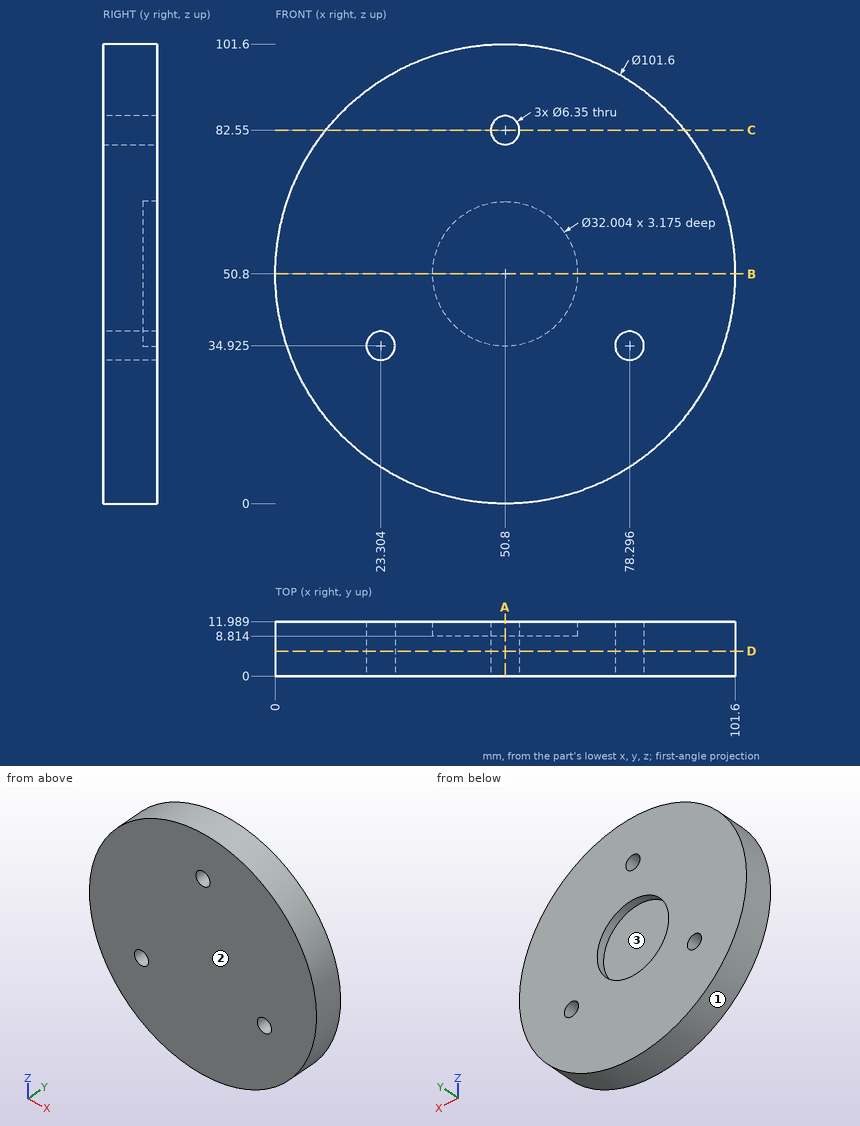
Geometry: see drawing. Coordinates: mm, zero at the bounding-box minimum. Give positions to 0.01 mm unless a question says otherwise; leave off trailing zeros. Order: outer loops, then holes, each group sorted by start corner. A loop starts at its lowest first (then second) coordinate and runs counter-clockwise, first axis right, second up. Notation, with made-up numbers: M -25.5,-8.5 L -13.5,-8.5 A13 ccw -13.5,10.5 Z; hole C 65.5,-8.5 d9. An arc over 180 degrees is marked long. Answer as a JSON object with one key per item and string values.
1. First-contact query: P1, Ø2, axis at x = 19.5, y = 6, coming from the -Z side (1 decimal); P2, Ø1.5, axis at x = 46, y = 3, coming from the -Z side; P3, Ø5.5, axis at x = 23.3, z = 34.92, coming from the +Y side (3 decimals); P4, Ø5, axis at x = 72, z = 45.5, coming from the -Y side. Flat tips, straight axial feed; report the tip coordinate or a pass-through.
Result sheet:
{"P1": "z = 10", "P2": "z = 0.16", "P3": "through", "P4": "y = 0"}
2. Pull-direction query (Z, two-part tool) for the marked faces 1, 2 and 3; classes: +Z half, -Z half, draft (parallel to the pull), parting line (faces both ways), or undercut.
Result sheet:
{"face 1": "parting line", "face 2": "draft", "face 3": "undercut"}
3. Cut plane B-B, the plane z = 50.8. Output: boundary loops of the cut face in (x, y).
Result sheet:
{"outline": "M 0,0 L 101.6,0 L 101.6,11.99 L 66.8,11.99 L 66.8,8.81 L 34.8,8.81 L 34.8,11.99 L 0,11.99 Z"}
4. Cut plane A-A, the plane x = 50.8. Output: boundary loops of the cut face in (y, z) (1 decimal), and give its area (3 significant figures).
Result sheet:
{"outline": "M 0,0 L 12,0 L 12,34.8 L 8.8,34.8 L 8.8,66.8 L 12,66.8 L 12,79.4 L 0,79.4 Z; M 0,85.7 L 12,85.7 L 12,101.6 L 0,101.6 Z", "area": "1,040 mm²"}
5. Ray query, line 1 (Y direction, x = 60.5, z = 45.5); line 2 (Z direction, x = 52, y = 10.5) (1 decimal); line 3 (X direction, y = 6.5, z = 84.5) (1 decimal). Return the intervals inside material, ascending. Write a range as [from, to].
Result sheet:
{"line 1": "[0, 8.81]", "line 2": "[0, 34.8], [66.8, 79.6], [85.5, 101.6]", "line 3": "[12.8, 48.3], [53.3, 88.8]"}
6. Cut plane C-C, the plane z = 82.55. Output: boundary loops of the cut face in (x, y) (1 decimal), and give its area (3 significant figures).
Result sheet:
{"outline": "M 11.1,0 L 47.6,0 L 47.6,12 L 11.1,12 Z; M 54,0 L 90.5,0 L 90.5,12 L 54,12 Z", "area": "875 mm²"}
7. Cut plane D-D, the plane y = 5.5. State how many separate pieces and enclosed holes the cut face has, and give its area (3 significant figures).
Result sheet:
{"separate pieces": "1", "enclosed holes": "3", "area": "8,010 mm²"}
